```python
from build123d import *

# Parameters (mm, degrees)
BOSS_EXTRUDE1_DEPTH   = 10.25
FILLET1_R             = 4
BOSS_EXTRUDE2_DEPTH   = 2
M5_CLEARANCE_HOLE1_D  = 5.5
M2X0_4_TAPPED_HOLE1_D = 1.6
FILLET2_R             = 1


with BuildPart() as part:
    # Sketch1 → Boss-Extrude1 (new, symmetric)
    with BuildSketch(Plane.XY):
        with BuildLine():
            Line((22, 4), (-22, 4))
            ThreePointArc((-22, 4), (-24.828427125, -2.828427125), (-18, 0))
            Line((-18, 0), (18, 0))
            ThreePointArc((18, 0), (24.828427125, -2.828427125), (22, 4))
        make_face()
    extrude(amount=BOSS_EXTRUDE1_DEPTH, both=True)

    # Fillet1
    fillet1_edges = [part.edges().sort_by_distance(p)[0] for p in [
        (18, 0, 0),
        (-18, 0, 0),
    ]]
    fillet(fillet1_edges, radius=FILLET1_R)

    # Sketch7 → Boss-Extrude2 (add)
    with BuildSketch(Plane.XZ.offset(-2)):
        Polygon((17, 10.25), (17, 18), (-17, 18), (-17, 10.25), (-15.07179677, 10.25), (15.07179677, 10.25), align=None)
    extrude(amount=-BOSS_EXTRUDE2_DEPTH)

    # M5 Clearance Hole1 (through all)
    with Locations(Plane.XY.offset(10.25)):
        with Locations((-22, 0), (22, 0)):
            Hole(M5_CLEARANCE_HOLE1_D / 2)

    # M2x0.4 Tapped Hole1 (through all)
    with Locations(Plane(origin=(0, 4, 0), x_dir=(1, 0, 0), z_dir=(0, 1, 0))):
        with Locations((14.25, 6.500000018), (14.25, -7.499999982), (-13.75, -7.499999982), (-13.75, 6.500000018)):
            Hole(M2X0_4_TAPPED_HOLE1_D / 2)

    # Fillet2
    fillet2_edges = [part.edges().sort_by_distance(p)[0] for p in [
        (17, 3, 18),
        (17, 3, 10.25),
        (-17, 3, 10.25),
        (-17, 3, 18),
    ]]
    fillet(fillet2_edges, radius=FILLET2_R)


solid = part.part
```
Read the model definition and answer for the solid it produces. Units are mm, in the model's axes. A direction names the side the tool comes from. Coordinates: 2 decimals unless noted, no trailing zeros. Loops run counter-clockwise (first coordinate to the right, second up) from the corner with the lowest first, then second, coordinate; pieces in that order, holes last. Notation, with made-up numbers: (8, 42) -> (48, 42) arc R29 cw to (48, 79) -> close; hole circle Ø1 at (8, -2). An arc over 180 degrees is marked (long way). Return JSON: item names as keys, results as strings.
Item 1: Flat-ended cylindrical pins translate along their axes: P1, Ø1, axis at y = 2.5, z = 13.5, coming from the +X side; P2, Ø2, axis at y = 3.5, z = 13.5, coming from the -X side; P3, Ø1.8, axis at x = 14.25, z = -6.5, coming from the -Y side; P4, Ø1.3, axis at x = 14.25, z = 7.5, coming from the -Y side. Find the tip coordinate at first contact, or state that the pin passes through.
Answers:
{"P1": "stops at x = 17", "P2": "stops at x = -17", "P3": "stops at y = 0", "P4": "passes through"}
Item 2: Find section A-A (z = -6.5). Count the separate pieces of the cut face and the enclosed holes in it, plus the area to 3 significant figures.
Answers:
{"separate pieces": "3", "enclosed holes": "2", "area": "194 mm2"}
Item 3: Find section C-C (x = -13.75). Determine the outline of the cut face in (y, z), plus the area to 3 significant figures.
Answers:
{"outline": "(0, -10.25) -> (4, -10.25) -> (4, -7.3) -> (0, -7.3) -> close; (0, -5.7) -> (4, -5.7) -> (4, 6.7) -> (0, 6.7) -> close; (0, 8.3) -> (4, 8.3) -> (4, 18) -> (2, 18) -> (2, 10.25) -> (0, 10.25) -> close", "area": "84.7 mm2"}
Item 4: For faces 1 (the flat face through (17, 3, 14)), 2 (the flat face through (0, 2, 14)), 3 (the flat face through (-17, 3, 14)), determine the directions among +Z, -Z, +X, -X, +Y, -Y from which every point of the face is accessible in a straight line to the end or side of a thin tool.
Answers:
{"face 1": "+Z, +X, +Y, -Y", "face 2": "+Z, +X, -X, -Y", "face 3": "+Z, -X, +Y, -Y"}
Item 5: Find section B-B (y = -1.25). Determine the outline of the cut face in (x, z), plus the area to 3 significant figures.
Answers:
{"outline": "(-25.8, -10.25) -> (-24.45, -10.25) -> (-24.45, 10.25) -> (-25.8, 10.25) -> close; (-19.55, -10.25) -> (-17.98, -10.25) -> (-17.98, 10.25) -> (-19.55, 10.25) -> close; (17.98, -10.25) -> (19.55, -10.25) -> (19.55, 10.25) -> (17.98, 10.25) -> close; (24.45, -10.25) -> (25.8, -10.25) -> (25.8, 10.25) -> (24.45, 10.25) -> close", "area": "120 mm2"}
Item 6: Find section D-D (x = -4). Determine the outline of the cut face in (y, z), plus the area to 3 significant figures.
Answers:
{"outline": "(0, -10.25) -> (4, -10.25) -> (4, 18) -> (2, 18) -> (2, 10.25) -> (0, 10.25) -> close", "area": "97.5 mm2"}
Item 7: For a pull along X with two mould halves and no side action, classify faces 4 (the cylindrical face through (-17.301, 3.014, 10.535)), 5 (the cylindrical face through (14.84, 1.97, -7.04)), 6 (the cylindrical face through (14.84, 1.97, 6.96)), 7 (the flat face through (0, 2, -10.25)) as +X half, -X half, draft (parallel to the pull), parting line (faces both ways), or undercut.
Answers:
{"face 4": "-X half", "face 5": "undercut", "face 6": "undercut", "face 7": "draft"}
Item 8: Find the intervals of material crossed by probe 1 along Z at (x, y) = (14.25, 2.7); probe 2 along X at (y, z) = (0.25, -8.5); probe 3 along Y at (x, z) = (-22, -2), in increasing order.
Answers:
{"probe 1": "z = -10.25 to -7.3, -5.7 to 6.7, 8.3 to 18", "probe 2": "x = -25.99 to -24.74, -19.26 to 19.26, 24.74 to 25.99", "probe 3": "y = -4 to -2.75, 2.75 to 4"}
